Input: part model. Units: mm. Frame: model coordinates. Give positions to 0.01 mm unless a question says otherwise; leave off trailing zeros. Loops run counter-clockwise (first coordinate to the right, second up) from the corner with the lowest first, then second, coordinate; pieces in that order, holes last. Notation, with made-up numbers: (1, 54.25) -> (8, 54.25) arc R18 cw to (8, 73.25) -> close; hole circle Ø11 at (6, 43.25). An arc over 180 degrees is marked (long way). Answer in a Markdown table with one row per item. Add a question column.
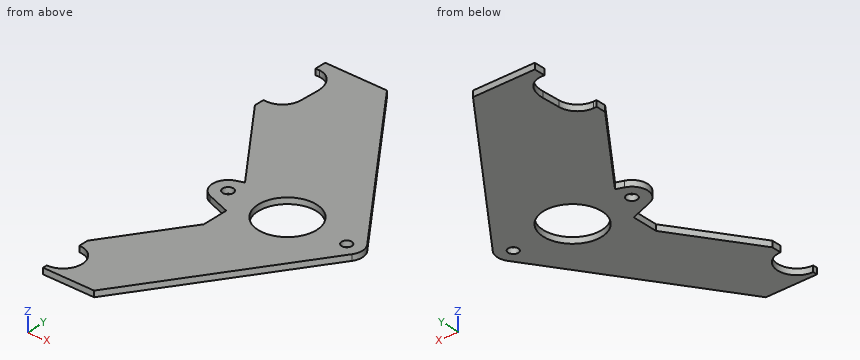
```python
from build123d import *

# Parameters (mm, degrees)
SKETCH1_R           = 3.565769245
SKETCH1_R_2         = 3.386490401
SKETCH1_R_3         = 19.5
BOSS_EXTRUDE1_DEPTH = 4
CUT_EXTRUDE1_DEPTH  = 4


with BuildPart() as part:
    # Sketch1 → Boss-Extrude1 (new body)
    with BuildSketch(Plane.XY):
        with BuildLine():
            ThreePointArc((-43.54375, 9.883918046), (-50.5, 0), (-43.54375, -9.883918046))
            Line((-43.54375, -9.883918046), (-27.881486705, -15.499418427))
            Line((-27.881486705, -15.499418427), (-27.881486705, -33.069179621))
            Line((-27.881486705, -33.069179621), (-62.35, -83.970607053))
            Line((-62.35, -83.970607053), (-62.35, -90.41))
            ThreePointArc((-62.35, -90.41), (-49.55, -103.21), (-62.35, -116.01))
            Line((-62.35, -116.01), (-62.35, -118.970607053))
            Line((-62.35, -118.970607053), (-27.881486705, -118.970607053))
            Line((-27.881486705, -118.970607053), (48.694184993, -5.887371851))
            ThreePointArc((48.694184993, -5.887371851), (50.496841017, 0.257543533), (48.395000292, 6.306660772))
            Line((48.395000292, 6.306660772), (-42.650294732, 127.5))
            Line((-42.650294732, 127.5), (-84.35, 127.5))
            Line((-84.35, 127.5), (-84.35, 72.5))
            Line((-84.35, 72.5), (-38.632989323, 11.644607286))
            Line((-38.632989323, 11.644607286), (-43.54375, 9.883918046))
        make_face()
        with Locations((-40, 0)):
            Circle(SKETCH1_R, mode=Mode.SUBTRACT)
        with Locations((40, 0)):
            Circle(SKETCH1_R_2, mode=Mode.SUBTRACT)
        Circle(SKETCH1_R_3, mode=Mode.SUBTRACT)
    extrude(amount=BOSS_EXTRUDE1_DEPTH)

    # Sketch2 → Cut-Extrude1 (cut)
    with BuildSketch(Plane(origin=(0, 0, 0), x_dir=(-1, 0, 0), z_dir=(0, 0, -1))):
        with BuildLine():
            Line((82.35, 79.081537598), (84.35, 79.081537598))
            Line((84.35, 79.081537598), (84.35, 119.944066118))
            Line((84.35, 119.944066118), (81.764527257, 119.944066118))
            add(Edge.make_bspline(
                [(69.254665804, 103.707956362), (68.93437366, 113.538092856), (74.471506462, 119.944066118), (81.764527257, 119.944066118)],
                knots=[0.236558718, 0.236558718, 0.236558718, 0.236558718, 1, 1, 1, 1], degree=3, weights=[0.82713852, 0.698801532, 0.756422025, 1]))
            Line((69.254665804, 103.707956362), (69.656735992, 91.3679571))
            ThreePointArc((69.656735992, 91.3679571), (73.517176905, 82.656230142), (82.35, 79.081537598))
        make_face()
    extrude(amount=-CUT_EXTRUDE1_DEPTH, mode=Mode.SUBTRACT)


solid = part.part
```
1) Material intervals for line 1 along Y through (x, z) = (-40, 2.75); line 2 along Y through (x, z) = (-60.5, 1.85); line 3 along Y through (x, z) = (0, 2.1), sorted ascending.
2) Pin query (flat end, axial travel): pin 1 (2 mm diameter, centred on x = -83, z = 2, fed in from -Y); pin 2 (1.2 mm diameter, centred on y = -88, z = 1, fed in from -X); pin 3 (5.5 mm diameter, centred on x = -40, y = 0, fed in from +Z). Return the tip coordinate at first contact, or that it passes through.
3) Section C-C on z = 2.15. State how many separate pieces and enclosed holes the cut face has, and give its area (3 significant figures).
4) Section D-D on x = -58. Output: boundary loops of the cut face in (y, z).
5) Section A-A on y = 0. Output: boundary loops of the cut face in (x, z), and give its area (3 significant figures).
6) Section B-B on x = 0. Output: boundary loops of the cut face in (y, z), and give its area (3 significant figures).
Working result:
| question | item | result |
|---|---|---|
| 1 | line 1 | y = -118.97 to -50.97, -11.15 to -3.57, 3.57 to 11.15, 13.46 to 123.97 |
| 1 | line 2 | y = -118.97 to -115.88, -90.54 to -81.24, 40.75 to 127.5 |
| 1 | line 3 | y = -77.8 to -19.5, 19.5 to 70.73 |
| 2 | pin 1 | stops at y = 69.37 |
| 2 | pin 2 | stops at x = -62.35 |
| 2 | pin 3 | passes through |
| 3 | separate pieces | 1 |
| 3 | enclosed holes | 3 |
| 3 | area | 14,700 mm2 |
| 4 | outline | (-118.97, 0) -> (-115.25, 0) -> (-115.25, 4) -> (-118.97, 4) -> close; (-91.17, 0) -> (-77.55, 0) -> (-77.55, 4) -> (-91.17, 4) -> close; (37.42, 0) -> (127.5, 0) -> (127.5, 4) -> (37.42, 4) -> close |
| 5 | outline | (-50.5, 0) -> (-43.57, 0) -> (-43.57, 4) -> (-50.5, 4) -> close; (-36.43, 0) -> (-19.5, 0) -> (-19.5, 4) -> (-36.43, 4) -> close; (19.5, 0) -> (36.61, 0) -> (36.61, 4) -> (19.5, 4) -> close; (43.39, 0) -> (50.5, 0) -> (50.5, 4) -> (43.39, 4) -> close |
| 5 | area | 192 mm2 |
| 6 | outline | (-77.8, 0) -> (-19.5, 0) -> (-19.5, 4) -> (-77.8, 4) -> close; (19.5, 0) -> (70.73, 0) -> (70.73, 4) -> (19.5, 4) -> close |
| 6 | area | 438 mm2 |
